Autodesk Fusion 360 part; units mm, degrees
sketch "Sketch1" plane through (0, 0, 0) normal (0, 0, 1) x (1, 0, 0)
  circle A0 centre (0, 0) radius 3 construction
  line L0 (12, 12) -> (-12, 12)
  line L1 (-12, 12) -> (-12, -12)
  line L2 (-12, -12) -> (12, -12)
  line L3 (12, -12) -> (12, 12)
  line L4 (12, 12) -> (-12, -12) construction
  line L5 (-12, 12) -> (12, -12) construction
  circle A1 centre (8, 8) radius 1.5 construction
  arc A2 (12, 8) -> (8, 12) centre (8, 8) ccw construction
  circle A3 centre (0, 0) radius 16 construction
  dimension "d1" = 6
  dimension "d2" = 24
  dimension "d3" = 3
  dimension "d4" = 8
  dimension "d23" = 32
extrude "Extrude1" add sketch "Sketch1" along normal blind 8
hole "Hole1" at (0, 0, 8) direction (0, 0, -1) diameter 6 end through all
sketch "Sketch2" plane through (0, 0, 8) normal (0, 0, 1) x (1, 0, 0)
  circle A0 centre (0, 0) radius 3
  line L0 (12, -12) -> (12, 12)
  line L1 (12, 12) -> (-12, 12)
  line L2 (-12, 12) -> (-12, -12)
  line L3 (-12, -12) -> (12, -12)
  line L4 (8, 8) -> (-8, 8)
  line L5 (-8, 8) -> (-8, -8)
  line L6 (-8, -8) -> (8, -8)
  line L7 (8, -8) -> (8, 8)
  line L8 (8, 8) -> (-8, -8) construction
  line L9 (-8, 8) -> (8, -8) construction
  dimension "d10" = 16
hole "Hole2" at (8, 8, 8) at (-8, 8, 8) at (-8, -8, 8) at (8, -8, 8) direction (0, 0, -1) diameter 3.332 end through all
sketch "Sketch3" plane through (0, 12, 0) normal (0, 1, 0) x (-1, 0, 0)
  line L0 (-12, 0) -> (12, 0)
  line L1 (12, 0) -> (12, 8)
  line L2 (12, 8) -> (-12, 8)
  line L3 (-12, 8) -> (-12, 0)
  line L4 (0, 0) -> (0, 8)
  line L5 (0, 4) -> (-12, 4)
hole "Hole3" at (0, 12, 4) direction (0, -1, 0) diameter 4.234 depth 10 tip angle 180
fillet "Fillet1" radius 4 4 edges at (12, 12, 4) (-12, 12, 4) (12, -12, 4) (-12, -12, 4)
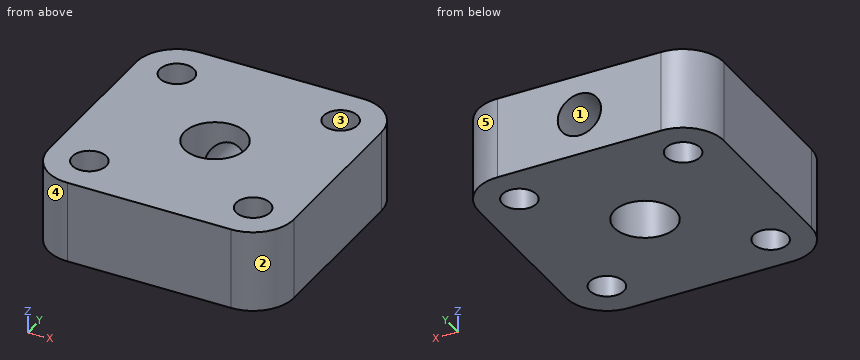
Verification items for the finished model (mm, model axes). Face numbers are marked on the shaded views. A direction names the side the tool comes from. Coordinates: 2 decimals unless noted, no trailing zeros. Order: outer loops, then holes, each group sorted by start corner. A loop starts at its lowest first (then second) coordinate and runs counter-clockwise, first axis right, second up. Notation, with made-up numbers: M -19,19.25 L 34,19.25 A20 ccw 34,50.25 Z; hole C 32.5,-38.75 d1. An arc over 180 degrees is marked long. Return JSON: item names as keys, results as strings.
1) Cross-section at C-C, the plane x = 1.25. Record the boundary of the cut face in (y, z), and give its area (3 significant figures).
Answer list:
{"outline": "M -12,0 L -2.73,0 L -2.73,8 L -12,8 Z; M 2.73,0 L 12,0 L 12,2.29 L 2.73,2.29 Z; M 2.73,5.71 L 12,5.71 L 12,8 L 2.73,8 Z", "area": "117 mm2"}
2) Cross-section at B-B, the plane y = 7.5. Record the boundary of the cut face in (x, z), and give its area (3 significant figures).
Answer list:
{"outline": "M -12,0 L -9.59,0 L -9.59,8 L -12,8 Z; M -6.41,0 L 6.41,0 L 6.41,8 L -6.41,8 Z; M 9.59,0 L 12,0 L 12,8 L 9.59,8 Z; hole C 0,4 d4.23", "area": "127 mm2"}
3) Access from +Z, -Z, +X, -X, +Y, -Y to the whole of each face (thin tool, end or side, straight path). Record for the marked faces 1 and 2.
Answer list:
{"face 1": "+Y", "face 2": "+Z, -Z, +X, -Y"}
4) Gauge pin test, flat end, axial feed: pin 1 (2 mm diameter, centred on x = 8, y = -8, fed in from -Z). Record the tip position at first contact, or that the pin passes through.
Answer list:
{"pin 1": "through"}
5) Release check for a two-part mould opening along Y. For the marked faces 3, 4 and 5 record: +Y half, -Y half, draft (parallel to the pull), parting line (faces both ways), or undercut.
Answer list:
{"face 3": "undercut", "face 4": "-Y half", "face 5": "+Y half"}
6) Cross-section at A-A, the plane y = 0. Record the boundary of the cut face in (x, z).
Answer list:
{"outline": "M -12,0 L -3,0 L -3,8 L -12,8 Z; M 3,0 L 12,0 L 12,8 L 3,8 Z"}
7) Cross-section at D-D, the plane z = 3.75. Record the boundary of the cut face in (x, y).
Answer list:
{"outline": "M -12,-8 A4 ccw -8,-12 L 8,-12 A4 ccw 12,-8 L 12,8 A4 ccw 8,12 L 2.1,12 L 2.1,2.14 A3 cw long -2.1,2.14 L -2.1,12 L -8,12 A4 ccw -12,8 Z; hole C -8,-8 d3.33; hole C -8,8 d3.33; hole C 8,-8 d3.33; hole C 8,8 d3.33"}
8) Thickness scan on L1, parallel to X at y = -8, z = 3.75; L2, parallel to X at y = 6, z = 4. Record the ranges inside material, lowest first. Write a range as [from, to].
Answer list:
{"L1": "[-12, -9.67], [-6.33, 6.33], [9.67, 12]", "L2": "[-12, -2.12], [2.12, 12]"}
